For this review, take the finished solid that the model builds, in its own axes (mm). A direction names the side the tool comes from. Round coordinates to 2 decimals unless told otherwise and drop trailing zeros. Order: outer loops, then holes, each group sorted by start corner. A loop starts at its lowest first (then second) coordinate and runs counter-clockwise, first axis right, second up. Notation, with made-up numbers: (60.25, 26.25) -> (64.25, 26.25) arc R15 cw to (64.25, 44.25) -> close; hole circle Ø11 at (74.25, 85). An arc over 180 degrees is marked (long way). Answer in a Markdown table with one row per item.
```python
from build123d import *

# Parameters (mm, degrees)
SKETCH1_R           = 1.5
BOSS_EXTRUDE4_DEPTH = 1.5
SKETCH1_7_R         = 3.5
SKETCH1_7_R_2       = 2.5
BOSS_EXTRUDE5_DEPTH = 3.8


with BuildPart() as part:
    # Sketch1 → Boss-Extrude4 (new body)
    with BuildSketch(Plane(origin=(0, 0, 0), x_dir=(1, 0, 0), z_dir=(0, 1, 0))):
        with BuildLine():
            Line((-29.654588032, -20.377951177), (-30.404588032, -32.212887668))
            ThreePointArc((-30.404588032, -32.212887668), (-27.654588032, -30.877951177), (-24.904588032, -32.212887668))
            Line((-24.904588032, -32.212887668), (-25.654588032, -20.377951177))
            ThreePointArc((-25.654588032, -20.377951177), (-27.654588032, -18.377951177), (-29.654588032, -20.377951177))
        make_face()
        with Locations(Location((-27.654588032, -21.545225809, 0), (0, 0, 270))):
            Circle(SKETCH1_R, mode=Mode.SUBTRACT)
    extrude(amount=BOSS_EXTRUDE4_DEPTH)

    # Sketch1_7 → Boss-Extrude5 (add)
    with BuildSketch(Plane(origin=(0, 0, 0), x_dir=(1, 0, 0), z_dir=(0, 1, 0))):
        with Locations(Location((-27.654588032, -34.377951177, 0), (0, 0, 38.213210702))):
            Circle(SKETCH1_7_R)
        with Locations(Location((-27.654588032, -34.377951177, 0), (0, 0, 90))):
            Circle(SKETCH1_7_R_2, mode=Mode.SUBTRACT)
    extrude(amount=BOSS_EXTRUDE5_DEPTH)


solid = part.part
```
Q1. Tool access review of faces 1 (the face through (-26.137, 1.873, 37.532)), 2 (the face through (-28, 0, 28)): name each direction out of +Z, -Z, +X, -X, +Y, -Y from which nothing blocks a thin tool from reaching the whole face with its end or side.
Answer key:
| item | result |
|---|---|
| face 1 | +Y |
| face 2 | +Z, -Z, +X, -X, -Y |
Q2. Clearance check with flat-ended pins moving along their axes: pin 1 Ø2 at (y, z) = (2, 22) entering from +X; pin 2 Ø1.5 at (x, z) = (-29.5, 33.5) entering from +Y; pin 3 Ø1 at (x, y) = (-25.5, 1.5) entering from +Z; pin 4 Ø1 at (y, z) = (1.5, 24) entering from -X. State where each tip first meets the part, or that it passes through.
Answer key:
| item | result |
|---|---|
| pin 1 | stops at x = -25.5 |
| pin 2 | stops at y = 3.8 |
| pin 3 | stops at z = 37.46 |
| pin 4 | stops at x = -29.92 |
Q3. The part is to be moulded in two halves that separate along X. For faces 3 (the face through (-30, 3.8, 33)), 4 (the face through (-27.61, 0.74, 18.38)), 5 (the face through (-26.167, 0.74, 21.35)), say which applies: +X half, -X half, draft (parallel to the pull), parting line (faces both ways), or undercut.
Answer key:
| item | result |
|---|---|
| face 3 | draft |
| face 4 | parting line |
| face 5 | undercut |
Q4. Take a section at A-A, the plane z = 34.75. Write out the cut boundary in (x, y), then the cut area to 3 significant figures.
Answer key:
| item | result |
|---|---|
| outline | (-31.13, 0) -> (-30.13, 0) -> (-30.13, 3.8) -> (-31.13, 3.8) -> close; (-25.18, 0) -> (-24.17, 0) -> (-24.17, 3.8) -> (-25.18, 3.8) -> close |
| area | 7.66 mm^2 |
Q5. Take a section at B-B, the plane x = -26.5. Write out the cut boundary in (y, z).
Answer key:
| item | result |
|---|---|
| outline | (0, 18.74) -> (1.5, 18.74) -> (1.5, 20.59) -> (0, 20.59) -> close; (0, 22.5) -> (1.5, 22.5) -> (1.5, 31.07) -> (3.8, 31.07) -> (3.8, 32.16) -> (0, 32.16) -> close; (0, 36.6) -> (3.8, 36.6) -> (3.8, 37.68) -> (0, 37.68) -> close |
Q6. To check wall thickness, follow probe 1 along Z at (x, y) = (-27.5, 3.35); probe 2 along Z at (x, y) = (-28.75, 0.55); probe 3 along Y at (x, z) = (-26.25, 27.25). State the ranges of each line that lie inside material, in increasing order.
Answer key:
| item | result |
|---|---|
| probe 1 | z = 30.88 to 31.88, 36.87 to 37.87 |
| probe 2 | z = 18.7 to 20.52, 22.57 to 32.13, 36.63 to 37.7 |
| probe 3 | y = 0 to 1.5 |
Q7. Take a section at D-D, the plane y = 0.65. Write out the cut boundary in (x, z), then the cut area to 3 significant figures.
Answer key:
| item | result |
|---|---|
| outline | (-30.4, 32.21) -> (-29.65, 20.38) arc R2 ccw to (-25.65, 20.38) -> (-24.9, 32.21) arc R3.5 ccw (long way) to start; hole circle Ø5 at (-27.65, 34.38); hole circle Ø3 at (-27.65, 21.55) |
| area | 69.2 mm^2 |
Q8. Take a section at C-C, the plane z = 22. Write out the cut boundary in (x, y).
Answer key:
| item | result |
|---|---|
| outline | (-29.76, 0) -> (-29.08, 0) -> (-29.08, 1.5) -> (-29.76, 1.5) -> close; (-26.23, 0) -> (-25.55, 0) -> (-25.55, 1.5) -> (-26.23, 1.5) -> close |
